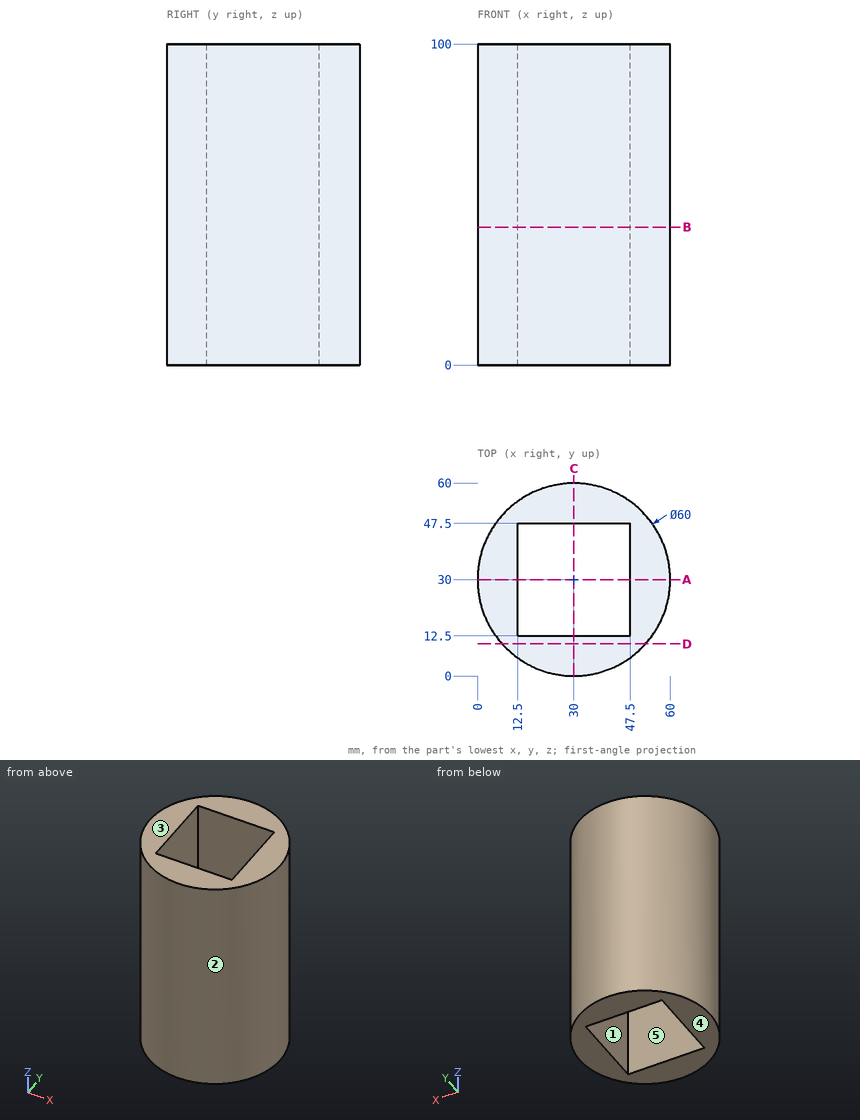
Job drawing, mm, ordinate dimensions from the low corner. One solid piece. A direction names the side the tool comes from. Give positions to 0.01 mm unless a question says otherwise; leave off trailing zeros. Loops run counter-clockwise (first coordinate to the right, second up) from the corner with the lowest first, then second, coordinate; pieces in that order, holes last. Notation, with made-up numbers: M 52.25,17.25 L 94.25,17.25 A10 cw 94.25,21.25 Z; hole C 53.25,70 d5. An arc over 180 degrees is marked long. Put each result on its own line as item: value. Start each with the question number.
1) Saw through at B-B (z = 43). List the corners of the cut face in (x, y), then the cut area to 3 significant figures.
2) Pull direction Y, two halves, no side cores. Call the marked faces 1, 2 and 3: +Y half, -Y half, draft (parallel to the pull), parting line (faces both ways), or undercut.
3) Saw through at D-D (y = 10). List the corners of the cut face in (x, z), then the cut area to 3 significant figures.
4) Probe probe 1 along X at (y, z) = (35.5, 91.5); probe 2 along X at (y, z) = (16, 68); probe 3 along Y at (x, z) = (32, 40). List the from-to ranges inside material, lowest first.
5) 3-axis set-ups, long thin cutter, end or side, ignore diameter. For the marked faces 4 and 5: which of +Z, -Z, +X, -X, +Y, -Y reach the whole face in a straight line?
6) Saw through at A-A (y = 30). List the corners of the cut face in (x, z).
7) Flat gauge pins, fed straight in: pin 1 (8 mm diameter, centred on x = 28.5, z = 52.5, fed in from +Y); pin 2 (5 mm diameter, centred on x = 46.5, z = 75, fed in from +Y); pin 3 (5 mm diameter, centred on x = 47, z = 83.5, fed in from -Y). Where does each tip first touch, or does it go through?
Numbers:
1. outline: C 30,30 d60; hole M 12.5,12.5 L 47.5,12.5 L 47.5,47.5 L 12.5,47.5 Z
1. area: 1,600 mm^2
2. face 1: undercut
2. face 2: parting line
2. face 3: draft
3. outline: M 7.64,0 L 52.36,0 L 52.36,100 L 7.64,100 Z
3. area: 4,470 mm^2
4. probe 1: 0.51 to 12.5, 47.5 to 59.49
4. probe 2: 3.47 to 12.5, 47.5 to 56.53
4. probe 3: 0.07 to 12.5, 47.5 to 59.93
5. face 4: -Z, +X, -X, +Y, -Y
5. face 5: +Z, -Z
6. outline: M 0,0 L 12.5,0 L 12.5,100 L 0,100 Z; M 47.5,0 L 60,0 L 60,100 L 47.5,100 Z
7. pin 1: y = 60
7. pin 2: y = 56.53
7. pin 3: y = 3.74
